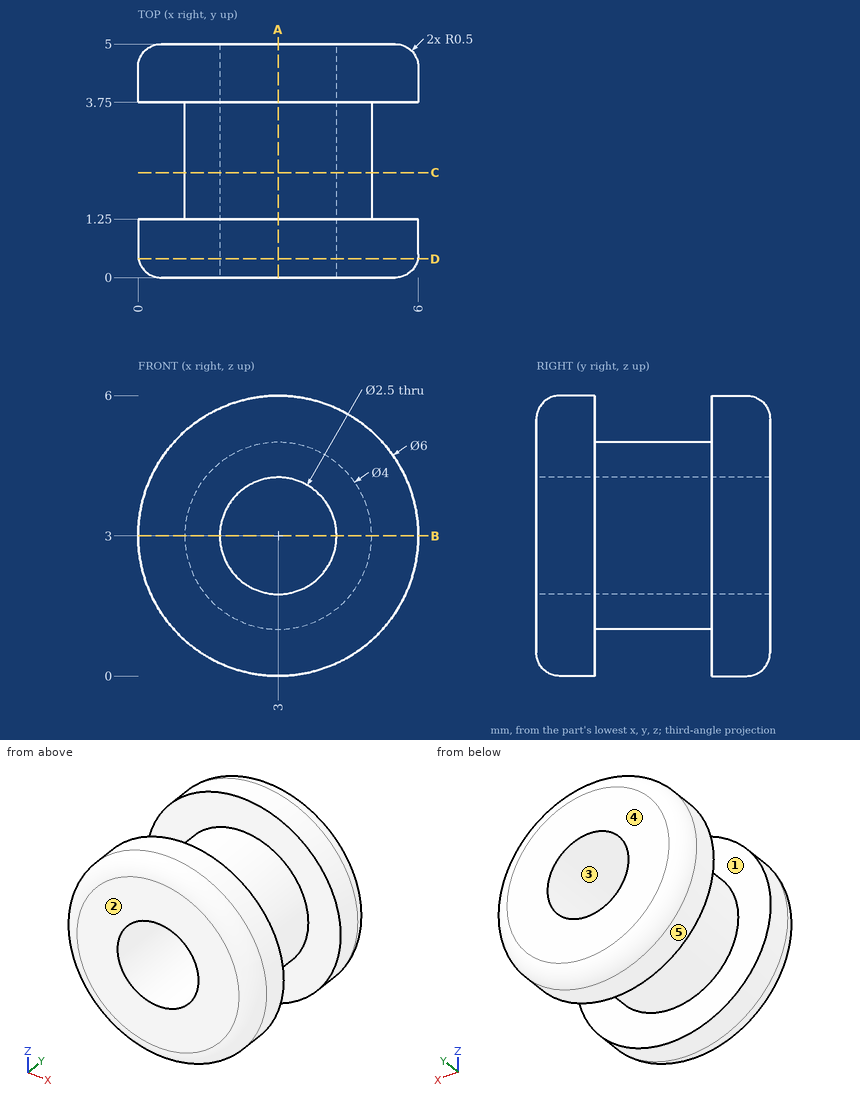
Job drawing, mm, ordinate dimensions from the low corner. One solid piece. A direction names the side the tool comes from. Round coordinates to 2 decimals unless told otherwise and drop trailing zeros. Loops run counter-clockwise (first coordinate to the right, second up) from the corner with the lowest first, then second, coordinate; pieces in that order, holes last.
Item 1: Cut at C-C, the plane y = 2.25. Give the cut face in (x, z), then the cut area to 3 significant figures.
Item 2: Mould opens along X. For the marked faces 3, 4 and 5 say: +X half, -X half, draft (parallel to the pull), parting line (faces both ways), or undercut.
Item 3: Drop a flat-ended pin along its axis: P1, Ø2, axis at x = 3, y = 3.5, coming from the -Z side. Give the stop position or say it passes through.
Item 4: Cut at B-B, the plane z = 3. Give the cut face in (x, y).
Item 5: 3-axis set-ups, long thin cutter, end or side, ignore diameter. For the marked faces 1 and 2: which of +Z, -Z, +X, -X, +Y, -Y reach the whole face in a straight line?
Item 6: Drill centre lines: line 1 (Z direction, x = 3, y = 3.65); line 2 (Y direction, x = 1.2, z = 4.35); line 3 (Y direction, x = 2.45, z = 0.3). Where is each one in solid material? Low to high.
Item 7: Cut at A-A, the plane x = 3. Give the cut face in (y, z).
Item 8: Cut at D-D, the plane y = 0.4. Give the cut face in (x, z).
A:
1. outline: circle Ø4 at (3, 3); hole circle Ø2.5 at (3, 3)
1. area: 7.66 mm2
2. face 3: undercut
2. face 4: draft
2. face 5: parting line
3. P1: stops at z = 0
4. outline: (0, 0.5) arc R0.5 ccw to (0.5, 0) - (1.75, 0) - (1.75, 5) - (0.5, 5) arc R0.5 ccw to (0, 4.5) - (0, 3.75) - (1, 3.75) - (1, 1.25) - (0, 1.25) - close; (4.25, 0) - (5.5, 0) arc R0.5 ccw to (6, 0.5) - (6, 1.25) - (5, 1.25) - (5, 3.75) - (6, 3.75) - (6, 4.5) arc R0.5 ccw to (5.5, 5) - (4.25, 5) - close
5. face 1: none
5. face 2: +Z, -Z, +X, -X, -Y
6. line 1: z = 1 to 1.75, 4.25 to 5
6. line 2: y = 0 to 1.25, 3.75 to 5
6. line 3: y = 0.07 to 1.25, 3.75 to 4.93
7. outline: (0, 0.5) arc R0.5 ccw to (0.5, 0) - (1.25, 0) - (1.25, 1) - (3.75, 1) - (3.75, 0) - (4.5, 0) arc R0.5 ccw to (5, 0.5) - (5, 1.75) - (0, 1.75) - close; (0, 4.25) - (5, 4.25) - (5, 5.5) arc R0.5 ccw to (4.5, 6) - (3.75, 6) - (3.75, 5) - (1.25, 5) - (1.25, 6) - (0.5, 6) arc R0.5 ccw to (0, 5.5) - close
8. outline: circle Ø5.98 at (3, 3); hole circle Ø2.5 at (3, 3)
